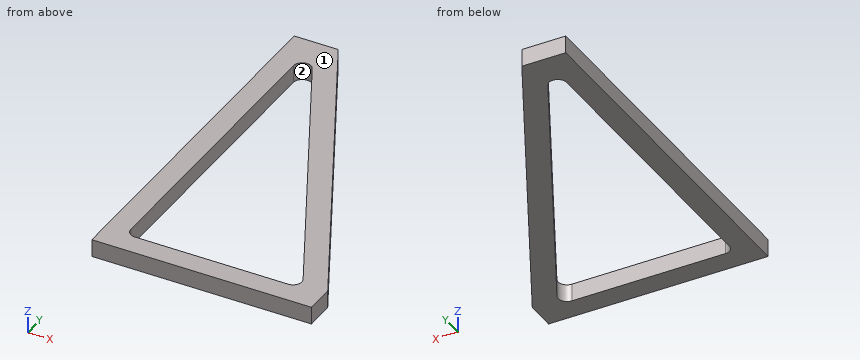
```python
from build123d import *

# Parameters (mm, degrees)
BOSS_EXTRUDE1_DEPTH = 12


with BuildPart() as part:
    # Sketch1 → Boss-Extrude1 (new body)
    with BuildSketch(Plane.XY):
        Polygon((150, 0), (0, 0), (0, 250), (30, 250), (150, 20), align=None)
        with BuildLine():
            Line((26.319509077, 224.626469841), (131.111373669, 23.77539604))
            ThreePointArc((131.111373669, 23.77539604), (130.922769787, 17.88972479), (125.791864592, 15))
            Line((125.791864592, 15), (21, 15))
            ThreePointArc((21, 15), (16.757359313, 16.757359313), (15, 21))
            Line((15, 21), (15, 221.851073801))
            ThreePointArc((15, 221.851073801), (19.571198835, 227.67846835), (26.319509077, 224.626469841))
        make_face(mode=Mode.SUBTRACT)
    extrude(amount=BOSS_EXTRUDE1_DEPTH)


solid = part.part
```
Work out the finished part from the listing and answer in its coordinate system (mm). Face numbers are marked on the shaded views. Coordinates: 2 decimals unless noted, no trailing zeros. Order: outer loops, then holes, each group sorted by start corner. A loop starts at its lowest first (then second) coordinate and runs counter-clockwise, first axis right, second up. Notation, with made-up numbers: M 31.5,26.5 L 68.5,26.5 A24 cw 68.5,46.5 Z; hole C 2,-34.75 d9. An arc over 180 degrees is marked long. Use CSV: the item, a comma, the result in double quotes.
1) Flat-ended cylindrical pins translate along their axes: pin 1 Ø3 at (y, z) = (38.5, 4) entering from +X; pin 2 Ø6 at (y, z) = (137, 4) entering from +X; pin 3 Ø6 at (x, z) = (51, 7) entering from +Y. Find the tip coordinate at first contact, or state that the pin passes through.
Worked out:
pin 1,"stops at x = 141.13"
pin 2,"stops at x = 90.52"
pin 3,"stops at y = 215.5"
2) Consider line 1 (Y direction, x = 18.5, z = 6); line 2 (X direction, y = 122.5, z = 3); line 3 (Y direction, x = 110, z = 3). Determine where each line is inside the solid, lowest interval first. Write a range as [from, to].
Worked out:
line 1,"y = [0, 15.55], [227.31, 250]"
line 2,"x = [0, 15], [79.6, 96.52]"
line 3,"y = [0, 15], [64.24, 96.67]"
3) Section D-D on x = 134.5 is taken. Write down the section's boundary in (y, z), plus the area to 4 significant figures.
Worked out:
outline,"M 0,0 L 49.71,0 L 49.71,12 L 0,12 Z"
area,"596.5 mm^2"
4) Section C-C on y = 29 is taken. Write down the section's boundary in (x, z), plus the area to 3 significant figures.
Worked out:
outline,"M 0,0 L 15,0 L 15,12 L 0,12 Z; M 128.39,0 L 145.3,0 L 145.3,12 L 128.39,12 Z"
area,"383 mm^2"
5) Determine the mould class of the marked faces 1 and 2 for opening direction Y: released by +Y, released by -Y, zero draft, split by the parting line, or undercut.
Worked out:
face 1,"zero draft"
face 2,"undercut"
6) Section B-B on x = 52 is taken. Write down the section's boundary in (y, z).
Worked out:
outline,"M 0,0 L 15,0 L 15,12 L 0,12 Z; M 175.41,0 L 207.83,0 L 207.83,12 L 175.41,12 Z"
7) Section A-A on z = 5.75 is taken. Write down the section's boundary in (x, y), plus the area to 3 significant figures.
Worked out:
outline,"M 0,0 L 150,0 L 150,20 L 30,250 L 0,250 Z; hole M 15,21 A6 ccw 21,15 L 125.79,15 A6 ccw 131.11,23.78 L 26.32,224.63 A6 ccw 15,221.85 Z"
area,"9,870 mm^2"
